```python
from build123d import *
from build123d.topology import SkipClean

# Parameters (mm, degrees)
SKETCH1_R                         = 34
BOSS_EXTRUDE1_DEPTH               = 2
M2_CLEARANCE_HOLE1_D              = 2.4
SKETCH11_W                        = 42
SKETCH11_H                        = 42
BOSS_EXTRUDE3_DEPTH               = 2
TAP_START                         = -2
TAP_DRILL_FOR_M2_5_TAP1_OUTLINE_R = 1.025
TAP_DRILL_FOR_M2_5_TAP1_DEPTH     = 4
CUT_EXTRUDE1_DEPTH                = 49.124837662
CUT_EXTRUDE1_DEPTH_BACK           = 2
SKETCH10_R                        = 1.6
SKETCH12_W                        = 39
SKETCH12_H                        = 39
CUT_EXTRUDE2_DEPTH                = 3
SKETCH13_R                        = 1.025
BOSS_EXTRUDE4_DEPTH               = 1
FILLET1_R                         = 1
FILLET2_R                         = 5
CUT_EXTRUDE3_DEPTH                = 49.176757882
BOSS_EXTRUDE5_START               = 2
BOSS_EXTRUDE5_DEPTH               = 2
FILLET3_R                         = 4
FILLET4_R                         = 2
FILLET5_R                         = 3
CUT_EXTRUDE4_DEPTH                = 49.124837662
CUT_EXTRUDE4_DEPTH_BACK           = 49.124837662
SKETCH16_W                        = 58.171472577
SKETCH16_H                        = 11
FILLET6_R                         = 5


# Read off the part's stored shape, not the designer's step: Tap Drill for M2.5 Tap1
with BuildPart() as part:
    # Sketch1 → Boss-Extrude1 (new body)
    with BuildSketch(Plane(origin=(0, 0, 0), x_dir=(1, 0, 0), z_dir=(0, 1, 0))):
        with Locations(Location((0, 0, 0), (0, 0, 270))):
            Circle(SKETCH1_R)
    extrude(amount=BOSS_EXTRUDE1_DEPTH)

    # M2 Clearance Hole1 (through all)
    with Locations(Plane(origin=(0, 2, 0), x_dir=(1, 0, 0), z_dir=(0, 1, 0))):
        with Locations((-23.815698604, -13.75), (0, 27.5), (23.815698604, -13.75)):
            Hole(M2_CLEARANCE_HOLE1_D / 2)

    # Sketch11 → Boss-Extrude3 (add)
    with BuildSketch(Plane.XZ):
        Rectangle(SKETCH11_W, SKETCH11_H)
    extrude(amount=BOSS_EXTRUDE3_DEPTH)

    # Tap Drill for M2.5 Tap1 outline → Tap Drill for M2.5 Tap1 (cut)
    with BuildSketch(Plane(origin=(0, 0, 0), x_dir=(1, 0, 0), z_dir=(0, 1, 0)).offset(TAP_START)):
        with Locations((-16, 16)):
            Circle(TAP_DRILL_FOR_M2_5_TAP1_OUTLINE_R)
        with Locations((16, -16)):
            Circle(TAP_DRILL_FOR_M2_5_TAP1_OUTLINE_R)
        with Locations((16, 16)):
            Circle(TAP_DRILL_FOR_M2_5_TAP1_OUTLINE_R)
        with Locations((-16, -16)):
            Circle(TAP_DRILL_FOR_M2_5_TAP1_OUTLINE_R)
    extrude(amount=TAP_DRILL_FOR_M2_5_TAP1_DEPTH, mode=Mode.SUBTRACT)

    # Sketch10 → Cut-Extrude1 (cut, two sides: drawn at the far end of the back side and taken through both)
    with BuildSketch(Plane.XZ.offset(-CUT_EXTRUDE1_DEPTH_BACK)):
        with Locations(Location((0, -27.5, 0), (0, 0, 90))):
            Circle(SKETCH10_R)
        with Locations(Location((-23.815698604, 13.75, 0), (0, 0, 90))):
            Circle(SKETCH10_R)
        with Locations(Location((23.815698604, 13.75, 0), (0, 0, 90))):
            Circle(SKETCH10_R)
    extrude(amount=CUT_EXTRUDE1_DEPTH + CUT_EXTRUDE1_DEPTH_BACK, mode=Mode.SUBTRACT)

    # Sketch12 → Cut-Extrude2 (cut)
    with BuildSketch(Plane(origin=(0, 2, 0), x_dir=(1, 0, 0), z_dir=(0, 1, 0))):
        Rectangle(SKETCH12_W, SKETCH12_H)
    extrude(amount=-CUT_EXTRUDE2_DEPTH, mode=Mode.SUBTRACT)

    # Sketch13 → Boss-Extrude4 (add)
    # profile 1 of 4: a face of its own
    with BuildSketch(Plane(origin=(0, -1, 0), x_dir=(1, 0, 0), z_dir=(0, 1, 0))):
        with BuildLine():
            Line((-12.5, 16), (-12.5, 19.5))
            Line((-12.5, 19.5), (-19.5, 19.5))
            Line((-19.5, 19.5), (-19.5, 12.5))
            Line((-19.5, 12.5), (-16, 12.5))
            ThreePointArc((-16, 12.5), (-13.525126266, 13.525126266), (-12.5, 16))
        make_face()
        with Locations(Location((-16, 16, 0), (0, 0, 270))):
            Circle(SKETCH13_R, mode=Mode.SUBTRACT)
    # profile 2 of 4: a face of its own
    with BuildSketch(Plane(origin=(0, -1, 0), x_dir=(1, 0, 0), z_dir=(0, 1, 0))):
        with BuildLine():
            Line((16, 12.5), (19.5, 12.5))
            Line((19.5, 12.5), (19.5, 19.5))
            Line((19.5, 19.5), (12.5, 19.5))
            Line((12.5, 19.5), (12.5, 16))
            ThreePointArc((12.5, 16), (13.525126266, 13.525126266), (16, 12.5))
        make_face()
        with Locations(Location((16, 16, 0), (0, 0, 270))):
            Circle(SKETCH13_R, mode=Mode.SUBTRACT)
    # profile 3 of 4: a face of its own
    with BuildSketch(Plane(origin=(0, -1, 0), x_dir=(1, 0, 0), z_dir=(0, 1, 0))):
        with BuildLine():
            Line((12.5, -16), (12.5, -19.5))
            Line((12.5, -19.5), (19.5, -19.5))
            Line((19.5, -19.5), (19.5, -12.5))
            Line((19.5, -12.5), (16, -12.5))
            ThreePointArc((16, -12.5), (13.525126266, -13.525126266), (12.5, -16))
        make_face()
        with Locations(Location((16, -16, 0), (0, 0, 270))):
            Circle(SKETCH13_R, mode=Mode.SUBTRACT)
    # profile 4 of 4: a face of its own
    with BuildSketch(Plane(origin=(0, -1, 0), x_dir=(1, 0, 0), z_dir=(0, 1, 0))):
        with BuildLine():
            Line((-16, -12.5), (-19.5, -12.5))
            Line((-19.5, -12.5), (-19.5, -19.5))
            Line((-19.5, -19.5), (-12.5, -19.5))
            Line((-12.5, -19.5), (-12.5, -16))
            ThreePointArc((-12.5, -16), (-13.525126266, -13.525126266), (-16, -12.5))
        make_face()
        with Locations(Location((-16, -16, 0), (0, 0, 270))):
            Circle(SKETCH13_R, mode=Mode.SUBTRACT)
    extrude(amount=BOSS_EXTRUDE4_DEPTH)

    # Fillet1
    fillet1_edges = [part.edges().sort_by_distance(p)[0] for p in [
        (-12.5, -0.5, -19.5),
        (-19.5, -0.5, -12.5),
        (19.5, -0.5, -12.5),
        (12.5, -0.5, -19.5),
        (12.5, -0.5, 19.5),
        (19.5, -0.5, 12.5),
        (-19.5, -0.5, 12.5),
        (-12.5, -0.5, 19.5),
    ]]
    fillet(fillet1_edges, radius=FILLET1_R)

    # Fillet2
    fillet2_edges = [part.edges().sort_by_distance(p)[0] for p in [
        (21, -1, -21),
        (21, -1, 21),
        (-21, -1, 21),
        (-21, -1, -21),
    ]]
    fillet(fillet2_edges, radius=FILLET2_R)

    # Sketch14 → Cut-Extrude3 (cut, through all)
    with BuildSketch(Plane(origin=(0, -1, 0), x_dir=(1, 0, 0), z_dir=(0, 1, 0))):
        with BuildLine():
            Line((12.5, 16), (12.5, 18.5))
            ThreePointArc((12.5, 18.5), (12.207106781, 19.207106781), (11.5, 19.5))
            Line((11.5, 19.5), (-11.5, 19.5))
            ThreePointArc((-11.5, 19.5), (-12.207106781, 19.207106781), (-12.5, 18.5))
            Line((-12.5, 18.5), (-12.5, 16))
            ThreePointArc((-12.5, 16), (-13.525126266, 13.525126266), (-16, 12.5))
            Line((-16, 12.5), (-18.5, 12.5))
            ThreePointArc((-18.5, 12.5), (-19.207106781, 12.207106781), (-19.5, 11.5))
            Line((-19.5, 11.5), (-19.5, -11.5))
            ThreePointArc((-19.5, -11.5), (-19.207106781, -12.207106781), (-18.5, -12.5))
            Line((-18.5, -12.5), (-16, -12.5))
            ThreePointArc((-16, -12.5), (-13.525126266, -13.525126266), (-12.5, -16))
            Line((-12.5, -16), (-12.5, -18.5))
            ThreePointArc((-12.5, -18.5), (-12.207106781, -19.207106781), (-11.5, -19.5))
            Line((-11.5, -19.5), (11.5, -19.5))
            ThreePointArc((11.5, -19.5), (12.207106781, -19.207106781), (12.5, -18.5))
            Line((12.5, -18.5), (12.5, -16))
            ThreePointArc((12.5, -16), (13.525126266, -13.525126266), (16, -12.5))
            Line((16, -12.5), (18.5, -12.5))
            ThreePointArc((18.5, -12.5), (19.207106781, -12.207106781), (19.5, -11.5))
            Line((19.5, -11.5), (19.5, 11.5))
            ThreePointArc((19.5, 11.5), (19.207106781, 12.207106781), (18.5, 12.5))
            Line((18.5, 12.5), (16, 12.5))
            ThreePointArc((16, 12.5), (13.525126266, 13.525126266), (12.5, 16))
        make_face()
    extrude(amount=-CUT_EXTRUDE3_DEPTH, mode=Mode.SUBTRACT)

    # Sketch15 → Boss-Extrude5 (add)
    with SkipClean():  # the faces are left unmerged after this step: merging them gives an invalid solid
        with BuildSketch(Plane.XZ.offset(BOSS_EXTRUDE5_START)):
            with BuildLine():
                Line((-10.145024857, 32.451170559), (-10.145024857, 21))
                Line((-10.145024857, 21), (10.145024857, 21))
                Line((10.145024857, 21), (10.145024857, 32.451170559))
                ThreePointArc((10.145024857, 32.451170559), (0, 34), (-10.145024857, 32.451170559))
            make_face()
            with BuildLine():
                Line((-21, 10.145024857), (-32.451170559, 10.145024857))
                ThreePointArc((-32.451170559, 10.145024857), (-34, 0), (-32.451170559, -10.145024857))
                Line((-32.451170559, -10.145024857), (-21, -10.145024857))
                Line((-21, -10.145024857), (-21, 10.145024857))
            make_face()
            with BuildLine():
                Line((-11, -21), (-11, -32.171415884))
                ThreePointArc((-11, -32.171415884), (-9.510045859, -32.642901644), (-8, -33.045423284))
                Line((-8, -33.045423284), (-8, -21))
                Line((-8, -21), (-11, -21))
            make_face()
            with BuildLine():
                ThreePointArc((8, -33.045423284), (9.510045859, -32.642901644), (11, -32.171415884))
                Line((11, -32.171415884), (11, -21))
                Line((11, -21), (8, -21))
                Line((8, -21), (8, -33.045423284))
            make_face()
            with BuildLine():
                ThreePointArc((34, 0), (33.610562321, 5.131286437), (32.451170559, 10.145024857))
                Line((32.451170559, 10.145024857), (21, 10.145024857))
                Line((21, 10.145024857), (21, -10.145024857))
                Line((21, -10.145024857), (32.451170559, -10.145024857))
                ThreePointArc((32.451170559, -10.145024857), (33.610562321, -5.131286437), (34, 0))
            make_face()
        extrude(amount=-BOSS_EXTRUDE5_DEPTH)

    # Fillet3
    fillet3_edges = [part.edges().sort_by_distance(p)[0] for p in [
        (-10.145024857, -1, 21),
        (10.145024857, -1, 21),
        (-21, -1, -10.145024857),
        (-21, -1, 10.145024857),
        (21, -1, 10.145024857),
        (21, -1, -10.145024857),
    ]]
    fillet(fillet3_edges, radius=FILLET3_R)

    # Fillet4
    fillet4_edges = [part.edges().sort_by_distance(p)[0] for p in [
        (-8, -1, -21),
        (-11, -1, -21),
        (11, -1, -21),
        (8, -1, -21),
    ]]
    fillet(fillet4_edges, radius=FILLET4_R)

    # Fillet5
    fillet5_edges = [part.edges().sort_by_distance(p)[0] for p in [
        (-19.5, 1, -19.5),
        (19.5, 1, -19.5),
        (19.5, 1, 19.5),
        (-19.5, 1, 19.5),
    ]]
    fillet(fillet5_edges, radius=FILLET5_R)

    # Sketch16 → Cut-Extrude4 (cut, two sides: drawn at the far end of the back side and taken through both)
    with SkipClean():  # the faces are left unmerged after this step: merging them gives an invalid solid
        with BuildSketch(Plane.XZ.offset(-CUT_EXTRUDE4_DEPTH_BACK)):
            with Locations((-0.899558855, 28.5)):
                Rectangle(SKETCH16_W, SKETCH16_H)
        extrude(amount=CUT_EXTRUDE4_DEPTH + CUT_EXTRUDE4_DEPTH_BACK, mode=Mode.SUBTRACT)

    # Fillet6
    fillet6_edges = [part.edges().sort_by_distance(p)[0] for p in [
        (10.680923241, -1, 23),
        (-25.039968051, 1, 23),
        (25.039968051, 1, 23),
        (-10.680923241, -1, 23),
    ]]
    fillet(fillet6_edges, radius=FILLET6_R)


solid = part.part
```
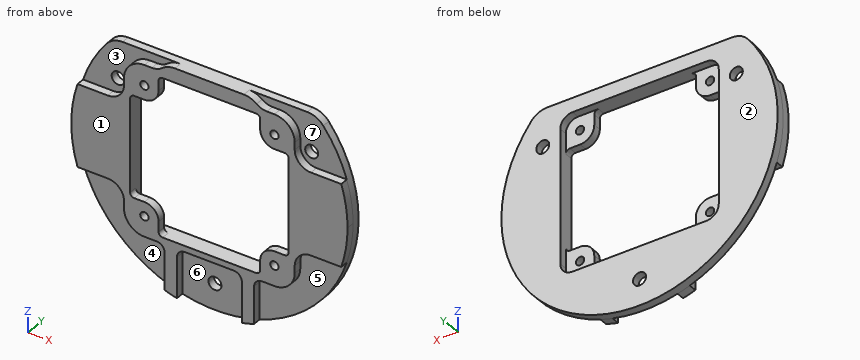
Geometry check sheet. Reference: the model listing, model coordinates, mm. Face numbers are marked on the shaded views. A direction names the side the tool comes from. Round coordinates to 2 decimals unless told otherwise and drop trailing zeros. Loops run counter-clockwise (first coordinate to the right, second up) from the corner with the lowest first, then second, coordinate; pieces in that order, holes last. Notation, with made-up numbers: (-8, -20) - (3, -20) arc R19 cw to (3, 16) - close; hole circle Ø4 at (-19.5, -17.75). An arc over 180 degrees is marked (long way). Write each question's results on one line, items separated by ' | '. Start each with the question number.
Q1. Access from +Z, -Z, +X, -X, +Y, -Y to the whole of each face (thin tool, end or side, straight path). Record for the marked faces 1, 2, 3, 4 and 5.
Q2. Cross-section at D-D on z = 8. Enter the section's corners in (x, y).
Q3. Cross-section at A-A on z = -1. Enter the section's corners in (x, y), and give its area (3 significant figures).
Q4. Release check for a two-part mould opening along X. For the marked faces 6 and 7 record: +X half, -X half, draft (parallel to the pull), parting line (faces both ways), or undercut.
Q5. Gauge pin test, flat ends, axial feed: P1, Ø1.5, axis at y = -1.5, z = -15, coming from the +X side; P2, Ø1.5, axis at y = -0.5, z = -3.5, coming from the -X side; P3, Ø1, axis at x = -30.5, y = -1, coming from the -Z side (3 decimals); P4, Ø17, axis at x = -18, z = -23, coming from the -Y side. Record the tip position at first contact, or that the pin passes through.
Q6. Cross-section at B-B on x = 3. Enter the section's corners in (y, z).
Q7. Thickness scan on line 1 (Z direction, x = 16, y = -0.9) (3 decimals); line 2 (X direction, y = -0.5, z = 0.5). Record the ranges inside material, lowest first. Write a range as [from, to].
Q8. Cross-section at C-C on x = 27.5. Enter the section's corners in (y, z).
Answers below:
1) face 1: +Z, -Z, +X, -X, -Y | face 2: +Z, -Z, +X, -X, +Y | face 3: +Z, -X, -Y | face 4: -Z, -X, -Y | face 5: -Z, +X, -Y
2) outline: (-33.05, -2) - (-19.5, -2) - (-19.5, 2) - (-33.05, 2) - close; (19.5, -2) - (33.05, -2) - (33.05, 2) - (19.5, 2) - close
3) outline: (-33.99, -2) - (-19.5, -2) - (-19.5, 2) - (-33.99, 2) - close; (19.5, -2) - (33.99, -2) - (33.99, 2) - (19.5, 2) - close | area: 116 mm²
4) face 6: undercut | face 7: draft
5) P1: stops at x = 21 | P2: stops at x = -33.89 | P3: stops at z = -10.145 | P4: stops at y = -2
6) outline: (-2, -21) - (0, -21) - (0, -33.87) - (2, -33.87) - (2, -19.5) - (-2, -19.5) - close; (-2, 19.5) - (2, 19.5) - (2, 23) - (-2, 23) - close
7) line 1: z = [-21, -17.025], [-14.975, -12.5], [12.5, 14.975], [17.025, 21] | line 2: x = [-34, -19.5], [19.5, 34]
8) outline: (-2, -10.15) - (0, -10.15) - (0, -19.99) - (2, -19.99) - (2, 19.99) - (0, 19.99) - (0, 10.15) - (-2, 10.15) - close
